```python
from build123d import *

# Parameters (mm, degrees)
EXTRUDE_2_DEPTH           = 3
SKETCH_4_R                = 2.25
SKETCH_4_R_2              = 2.5
CUT_EXTRUDE_2_DEPTH       = 96.402519291
SKETCH_6_R                = 3.5
CUT_EXTRUDE_3_DEPTH       = 96.402519291
SKETCH_7_R                = 3.5
CUT_EXTRUDE_4_DEPTH       = 96.402519291
CUT_EXTRUDE_5_DEPTH       = 96.402519291
EXTRUDE_4_DEPTH           = 15
EXTRUDE_5_DEPTH           = 3
SKETCH_11_R               = 4.1
CUT_EXTRUDE_6_DEPTH       = 3
SKETCH_13_R               = 3.5
EXTRUDE_6_DEPTH           = 3
SKETCH_14_R               = 2.05
EXTRUDE_7_DEPTH           = 5
EXTRUDE_START             = -5
SKETCH_15_R               = 4
SKETCH_15_R_2             = 2.05
EXTRUDE_8_DEPTH           = 5
CUT_EXTRUDE_7_DEPTH       = 96.878259721
SKETCH_18_R               = 1.397318861
CUT_EXTRUDE_8_DEPTH       = 144.753442506
CUT_EXTRUDE_9_DEPTH       = 97.527927136
CUT_EXTRUDE_9_DEPTH_BACK  = 97.527927136
CUT_EXTRUDE_11_DEPTH      = 110.140706759
CUT_EXTRUDE_11_DEPTH_BACK = 110.140706759
SKETCH_20_W               = 92.736362136
SKETCH_20_H               = 2.6
SKETCH_20_H_2             = 2.5
CUT_EXTRUDE_12_DEPTH      = 5


with BuildPart() as part:
    # 草图2 → 凸台-拉伸2 (new body)
    with BuildSketch(Plane(origin=(0, 0, 0), x_dir=(1, 0, 0), z_dir=(0, 1, 0))):
        with BuildLine():
            Line((-58.569449541, 23.337085947), (32.740581269, -53.879999426))
            ThreePointArc((32.740581269, -53.879999426), (53.033008589, -53.033008589), (53.879999426, -32.740581269))
            Line((53.879999426, -32.740581269), (-23.337085947, 58.569449541))
            ThreePointArc((-23.337085947, 58.569449541), (-60.104076401, 60.104076401), (-58.569449541, 23.337085947))
        make_face()
    extrude(amount=EXTRUDE_2_DEPTH)

    # 草图4 → 切除-拉伸2 (cut, through all)
    with BuildSketch(Plane(origin=(0, 3, 0), x_dir=(1, 0, 0), z_dir=(0, 1, 0))):
        with Locations(Location((-42.426406871, 42.426406871, 0), (0, 0, 270))):
            Circle(SKETCH_4_R)
        with Locations(Location((42.426406871, -42.426406871, 0), (0, 0, 270))):
            Circle(SKETCH_4_R_2)
    extrude(amount=-CUT_EXTRUDE_2_DEPTH, mode=Mode.SUBTRACT)

    # 草图6 → 切除-拉伸3 (cut, through all)
    with BuildSketch(Plane(origin=(0, 3, 0), x_dir=(1, 0, 0), z_dir=(0, 1, 0))):
        with Locations(Location((-42.426406871, 42.426406871, 0), (0, 0, 270))):
            Circle(SKETCH_6_R)
    extrude(amount=-CUT_EXTRUDE_3_DEPTH, mode=Mode.SUBTRACT)

    # 草图7 → 切除-拉伸4 (cut, through all)
    with BuildSketch(Plane(origin=(0, 3, 0), x_dir=(1, 0, 0), z_dir=(0, 1, 0))):
        with Locations(Location((42.426406871, -42.426406871, 0), (0, 0, 270))):
            Circle(SKETCH_7_R)
    extrude(amount=-CUT_EXTRUDE_4_DEPTH, mode=Mode.SUBTRACT)

    # 草图8 → 切除-拉伸5 (cut, through all)
    with BuildSketch(Plane(origin=(0, 3, 0), x_dir=(1, 0, 0), z_dir=(0, 1, 0))):
        Polygon((33.626672858, -22.564710472), (-15.702999665, 25.870376375), (-26.891422763, 12.98046534), (25.218843822, -32.251166492), align=None)
    extrude(amount=-CUT_EXTRUDE_5_DEPTH, mode=Mode.SUBTRACT)

    # 草图9 → 凸台-拉伸4 (add)
    with BuildSketch(Plane(origin=(0, 3, 0), x_dir=(1, 0, 0), z_dir=(0, 1, 0))):
        with BuildLine():
            ThreePointArc((-17.960284018, 47.565359346), (-19.96440182, 53.401757848), (-23.337085947, 58.569449541))
            ThreePointArc((-23.337085947, 58.569449541), (-60.104076401, 60.104076401), (-58.569449541, 23.337085947))
            ThreePointArc((-58.569449541, 23.337085947), (-53.401757848, 19.96440182), (-47.565359346, 17.960284018))
            Line((-47.565359346, 17.960284018), (-56.632284421, 25.627804458))
            ThreePointArc((-56.632284421, 25.627804458), (-57.982756057, 57.982756057), (-25.627804458, 56.632284421))
            Line((-25.627804458, 56.632284421), (-17.960284018, 47.565359346))
        make_face()
        with BuildLine():
            Line((53.879999426, -32.740581269), (-23.337085947, 58.569449541))
            ThreePointArc((-23.337085947, 58.569449541), (-19.96440182, 53.401757848), (-17.960284018, 47.565359346))
            Line((-17.960284018, 47.565359346), (45.777785554, -27.805590857))
            ThreePointArc((45.777785554, -27.805590857), (50.229311839, -29.615681908), (53.879999426, -32.740581269))
        make_face()
        with BuildLine():
            ThreePointArc((-47.565359346, 17.960284018), (-53.401757848, 19.96440182), (-58.569449541, 23.337085947))
            Line((-58.569449541, 23.337085947), (32.740581269, -53.879999426))
            ThreePointArc((32.740581269, -53.879999426), (29.615681908, -50.229311839), (27.805590857, -45.777785554))
            Line((27.805590857, -45.777785554), (-47.565359346, 17.960284018))
        make_face()
        with BuildLine():
            ThreePointArc((57.426406871, -42.426406871), (56.511929373, -37.26907657), (53.879999426, -32.740581269))
            ThreePointArc((53.879999426, -32.740581269), (50.229311839, -29.615681908), (45.777785554, -27.805590857))
            Line((45.777785554, -27.805590857), (51.589280915, -34.67774639))
            ThreePointArc((51.589280915, -34.67774639), (53.694824873, -38.30054263), (54.426406871, -42.426406871))
            ThreePointArc((54.426406871, -42.426406871), (47.47695507, -53.311808237), (34.67774639, -51.589280915))
            Line((34.67774639, -51.589280915), (27.805590857, -45.777785554))
            ThreePointArc((27.805590857, -45.777785554), (29.615681908, -50.229311839), (32.740581269, -53.879999426))
            ThreePointArc((32.740581269, -53.879999426), (48.73959212, -56.033158578), (57.426406871, -42.426406871))
        make_face()
    extrude(amount=EXTRUDE_4_DEPTH)

    # 草图10 → 凸台-拉伸5 (add)
    with BuildSketch(Plane(origin=(0, 3, 0), x_dir=(1, 0, 0), z_dir=(0, 1, 0))):
        Polygon((10.528753113, -10.528753113), (-20.427450775, 20.427450775), (-26.891422763, 12.98046534), (25.218843822, -32.251166492), (28.486536718, -28.486536718), align=None)
        Polygon((-15.702999665, 25.870376375), (-20.427450775, 20.427450775), (10.528753113, -10.528753113), (28.486536718, -28.486536718), (33.626672858, -22.564710472), align=None)
    extrude(amount=-EXTRUDE_5_DEPTH)

    # 草图11 → 切除-拉伸6 (cut)
    with BuildSketch(Plane(origin=(0, 3, 0), x_dir=(1, 0, 0), z_dir=(0, 1, 0))):
        with Locations(Location((-21.213203436, 21.213203436, 0), (0, 0, 270))):
            Circle(SKETCH_11_R)
    extrude(amount=-CUT_EXTRUDE_6_DEPTH, mode=Mode.SUBTRACT)

    # 草图13 → 凸台-拉伸6 (add)
    with BuildSketch(Plane(origin=(0, 3, 0), x_dir=(1, 0, 0), z_dir=(0, 1, 0))):
        with Locations((-42.426406871, 42.426406871)):
            Circle(SKETCH_13_R)
    extrude(amount=-EXTRUDE_6_DEPTH)

    # 草图14 → 凸台-拉伸7 (add)
    with BuildSketch(Plane(origin=(0, 3, 0), x_dir=(1, 0, 0), z_dir=(0, 1, 0))):
        with Locations(Location((-42.426406871, 42.426406871, 0), (0, 0, 270))):
            Circle(SKETCH_14_R)
    extrude(amount=EXTRUDE_7_DEPTH)

    # 草图15 → 凸台-拉伸8 (add)
    with BuildSketch(Plane(origin=(0, 8, 0), x_dir=(1, 0, 0), z_dir=(0, 1, 0)).offset(EXTRUDE_START)):
        with Locations(Location((-42.426406871, 42.426406871, 0), (0, 0, 270))):
            Circle(SKETCH_15_R)
        with Locations((-42.426406871, 42.426406871)):
            Circle(SKETCH_15_R_2, mode=Mode.SUBTRACT)
    extrude(amount=EXTRUDE_8_DEPTH)

    # 草图17 → 切除-拉伸7 (cut, through all)
    with BuildSketch(Plane(origin=(0, 8, 0), x_dir=(1, 0, 0), z_dir=(0, 1, 0))):
        with BuildLine():
            Line((-42.409215342, 44.476334785), (-43.439595085, 43.532503451))
            Line((-43.439595085, 43.532503451), (-44.469974827, 42.588672118))
            ThreePointArc((-44.469974827, 42.588672118), (-42.507603209, 40.378015513), (-40.376406871, 42.426406871))
            ThreePointArc((-40.376406871, 42.426406871), (-40.970772536, 43.869884853), (-42.409215342, 44.476334785))
        make_face()
    extrude(amount=-CUT_EXTRUDE_7_DEPTH, mode=Mode.SUBTRACT)

    # 草图18 → 切除-拉伸8 (cut, through all)
    with BuildSketch(Plane(origin=(-41.501827845, 0, -45.307504805), x_dir=(0.7373977200215518, 0, -0.6754588088899406), z_dir=(0.6754588088899406, 0, 0.7373977200215518))):
        with Locations((-2.627845445, 4.953208644)):
            Circle(SKETCH_18_R)
    extrude(amount=-CUT_EXTRUDE_8_DEPTH, mode=Mode.SUBTRACT)

    # 草图19 → 切除-拉伸9 (cut, two sides: drawn at the far end of the back side and taken through both)
    with BuildSketch(Plane(origin=(0, 3, 0), x_dir=(1, 0, 0), z_dir=(0, 1, 0)).offset(-CUT_EXTRUDE_9_DEPTH_BACK)):
        with BuildLine():
            Line((-66.29326799, 34.985107232), (-63.429244656, 35.878063189))
            ThreePointArc((-63.429244656, 35.878063189), (-57.900931168, 58.064152802), (-35.65805893, 63.35938244))
            Line((-35.65805893, 63.35938244), (-34.735102393, 66.213879108))
            ThreePointArc((-34.735102393, 66.213879108), (-60.011093572, 60.196572701), (-66.29326799, 34.985107232))
        make_face()
    extrude(amount=CUT_EXTRUDE_9_DEPTH + CUT_EXTRUDE_9_DEPTH_BACK, mode=Mode.SUBTRACT)

    # 草图20 → 切除-拉伸11 (cut, two sides: drawn at the far end of the back side and taken through both)
    with BuildSketch(Plane(origin=(-12.914434136, 0, 15.27145674), x_dir=(0.7635728369858691, 0, 0.6457217067881111), z_dir=(-0.6457217067881111, 0, 0.7635728369858691)).offset(-CUT_EXTRUDE_11_DEPTH_BACK)):
        with Locations((13.423122648, 10.3)):
            Rectangle(SKETCH_20_W, SKETCH_20_H)
        with Locations((13.423122648, 7.75)):
            Rectangle(SKETCH_20_W, SKETCH_20_H_2)
    extrude(amount=CUT_EXTRUDE_11_DEPTH + CUT_EXTRUDE_11_DEPTH_BACK, mode=Mode.SUBTRACT)

    # 草图23 → 切除-拉伸12 (cut)
    with BuildSketch(Plane(origin=(0, 3, 0), x_dir=(1, 0, 0), z_dir=(0, 1, 0))):
        Polygon((-34.648232278, 34.648232278), (-31.112698372, 31.112698372), (-24.04163056, 38.183766184), (-27.577164466, 41.71930009), align=None)
        Polygon((-38.192264962, 24.033131782), (-31.112698372, 31.112698372), (-34.648232278, 34.648232278), (-41.71930009, 27.577164466), align=None)
    extrude(amount=-CUT_EXTRUDE_12_DEPTH, mode=Mode.SUBTRACT)


solid = part.part
```
Geometry check sheet. Reference: the model listing, model coordinates, mm. A direction names the side the tool comes from. Give positions to 0.01 mm unless a question says otherwise; leave off trailing zeros. Loops run counter-clockwise (first coordinate to the right, second up) from the corner with the lowest first, then second, coordinate; pieces in that order, holes last. Notation, with made-up numbers: M -4,18.5 L 36,18.5 A26 cw 36,42.5 Z; hole C 14,-37 d1. An arc over 180 degrees is marked long. Write item = value, one per line. Start each with the question number.
1. Section check D-D, the plane y = 15.5. Enter the section's corners in (x, z), plus the area to 3 significant figures.
2. Draft check along Z on faces 1 (the face through (-41.225, 5.465, -38.611)), 2 (the face through (-63.317, 8.874, -28.693)), 3 (the face through (-28.421, 8.874, -63.135)). Enter one of: +Z half, -Z half, draft (parallel to the pull), parting line (faces both ways), or undercut.
3. Section check A-A, the plane x = 48. Enter the section's corners in (y, z).
4. Thickness scan on probe 1 along Y at (x, z) = (-7, -25); probe 2 along Z at (x, y) = (46, 12); probe 3 along X at (y, z) = (5.5, 33). Record the ranges inside material, lowest first.
5. Section check B-B, the plane z = -20. Enter the section's corners in (x, y).
6. Go/stop test with flat-tipped pins: P1, Ø1.5, axis at x = -23.5, y = 2.5, coming from the -Z side; P2, Ø6, axis at y = 12, z = -6, coming from the +X side; P3, Ø1.5, axis at y = 11.5, z = -6, coming from the -X side. Record where each tip stops, or that it passes through.
7. Tool access check on faces 4 (the face through (-5, 3, -5)), 5 (the face through (-60.713, 10.395, -30.196)), 6 (the face through (-34.549, 1.521, -34.747)). Record the directions out of +Z, -Z, +X, -X, +Y, -Y that give a thin tool (end or side, any length) a straight path to the whole face; none if there is none.
8. Section check C-C, the plane z = 49. Enter the section's corners in (x, y), plus the area to 3 significant figures.
Values follow:
q1.outline = M -66.29,-34.99 L -63.43,-35.88 A22 cw -56.63,-25.63 L 34.68,51.59 A12 cw 51.59,34.68 L -25.63,-56.63 A22 cw -35.66,-63.36 L -34.74,-66.21 A25 ccw -23.34,-58.57 L 53.88,32.74 A15 ccw 32.74,53.88 L -58.57,-23.34 A25 ccw Z
q1.area = 917 mm^2
q2.face_1 = undercut
q2.face_2 = +Z half
q2.face_3 = -Z half
q3.outline = M 0,25.79 L 6.5,25.79 L 6.5,30.43 L 3,30.43 L 3,53.05 L 18,53.05 L 18,56.35 L 0,56.35 Z; M 11.6,25.79 L 18,25.79 L 18,30.43 L 11.6,30.43 Z
q4.probe_1 = 0 to 3
q4.probe_2 = 23.42 to 28.07, 53.88 to 56.99
q4.probe_3 = 8.05 to 12.7, 50.17 to 54.09
q5.outline = M -54.62,0 L -25.13,0 L -25.13,3 L -49.98,3 L -49.98,18 L -54.62,18 Z; M -17.3,0 L 9.28,0 L 9.28,6.5 L 5.35,6.5 L 5.35,3 L -17.3,3 Z; M 5.35,11.6 L 9.28,11.6 L 9.28,18 L 5.35,18 Z
q6.P1 = -59.59
q6.P2 = 23.66
q6.P3 = -38.96
q7.face_4 = +Y
q7.face_5 = -Z, +Y
q7.face_6 = +Y, -Y
q8.outline = M 26.97,0 L 55.91,0 L 55.91,18 L 52.47,18 L 52.47,3 L 31.62,3 L 31.62,6.5 L 26.97,6.5 Z; M 26.97,11.6 L 31.62,11.6 L 31.62,18 L 26.97,18 Z
q8.area = 184 mm^2
